from build123d import *

# Parameters (mm, degrees)
BOSS_EXTRUDE2_DEPTH     = 35
SKETCH2_R               = 11
CUT_EXTRUDE1_DEPTH      = 35
SKETCH3_R               = 1.4605
CUT_EXTRUDE2_DEPTH      = 4.064
CUT_EXTRUDE3_REACH      = 55.991
CUT_EXTRUDE3_END_RADIUS = 11
SKETCH4_R               = 1.4605
LPATTERN1_COUNT         = 7
LPATTERN1_PITCH         = 3.5


with BuildPart() as part:
    # Sketch1 → Boss-Extrude2 (new body)
    with BuildSketch(Plane.XY):
        with BuildLine():
            Line((-12.177746097, -15.45), (-5.620498199, 2.1))
            ThreePointArc((-5.620498199, 2.1), (0, 6), (5.620498199, 2.1))
            Line((5.620498199, 2.1), (12.177746097, -15.45))
            ThreePointArc((12.177746097, -15.45), (0, -33), (-12.177746097, -15.45))
        make_face()
    extrude(amount=-BOSS_EXTRUDE2_DEPTH)

    # Sketch2 → Cut-Extrude1 (cut)
    with BuildSketch(Plane.XY):
        with Locations((0, -20)):
            Circle(SKETCH2_R)
    extrude(amount=-CUT_EXTRUDE1_DEPTH, mode=Mode.SUBTRACT)

    # Sketch3 → Cut-Extrude2 (cut)
    with BuildSketch(Plane.XY):
        with Locations((0, -9)):
            Circle(SKETCH3_R)
    extrude(amount=-CUT_EXTRUDE2_DEPTH, mode=Mode.SUBTRACT)

    # Cut-Extrude3: up to this cylinder (the profile starts outside it)
    cut_extrude3_end = Plane(origin=(0, -20, -32.5), z_dir=(0, 0, 1)) * Cylinder(CUT_EXTRUDE3_END_RADIUS, 134.982, mode=Mode.PRIVATE)
    # Sketch4 → Cut-Extrude3 (cut, up to the surface)
    with BuildSketch(Plane(origin=(0, 6, 0), x_dir=(1, 0, 0), z_dir=(0, 1, 0)), mode=Mode.PRIVATE) as cut_extrude3_sk1:
        with Locations(Location((0, 32.5, 0), (0, 0, 270))):
            Circle(SKETCH4_R)
    cut_extrude3_tool1 = extrude(cut_extrude3_sk1.sketch, amount=-CUT_EXTRUDE3_REACH, mode=Mode.PRIVATE) - cut_extrude3_end
    cut_extrude3 = cut_extrude3_tool1.solids().sort_by_distance((0, 6, -32.5))[0]
    add(cut_extrude3, mode=Mode.SUBTRACT)

    # LPattern1: Cut-Extrude3 ×7
    with Locations(*[(0, 0, i * LPATTERN1_PITCH) for i in range(1, LPATTERN1_COUNT)]):
        add(cut_extrude3, mode=Mode.SUBTRACT)


solid = part.part
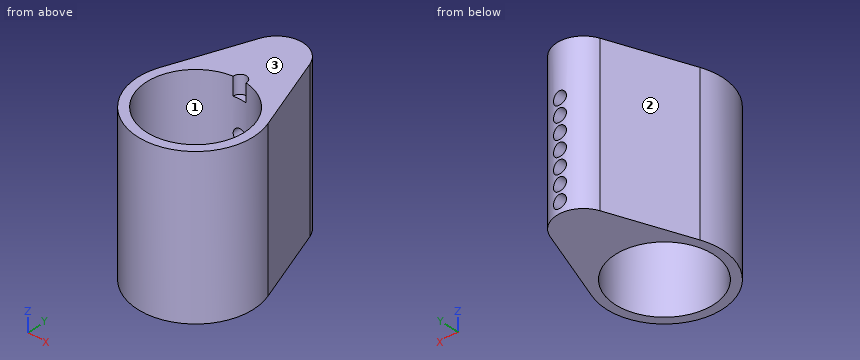
The listing builds one solid part. Answer for the finished solid, in the listing's coordinates (mm). Face numbers are marked on the shaded views. Coordinates: 2 decimals unless noted, no trailing zeros. Order: outer loops, then holes, each group sorted by start corner. A loop starts at its lowest first (then second) coordinate and runs counter-clockwise, first axis right, second up. Notation, with made-up numbers: M -15,-29.5 L 13,-29.5 A17 ccw 13,-5.5 Z; hole C 16.25,13.5 d4. An arc over 180 degrees is marked long. Use CSV: the item, a comma, the result in double quotes.
Q1. Given pin 1 Ø5 at (x, z) = (-3.5, -22.5) entering from +Y; pin 2 Ø2.5 at (x, z) = (0, -29) entering from +Y; pin 3 Ø1.8 at (x, z) = (0, -18.5) entering from +Y; pin 4 Ø3.5 at (x, z) = (0, -32.5) entering from +Y, each flat-ended and moving along its own axis, determine where each tip first touches the part or whether it passes through.
Here are the results:
pin 1,"y = 5.91"
pin 2,"y = -30.93"
pin 3,"y = -30.96"
pin 4,"y = 6"
Q2. Section B-B (x = -10) is taken. Determine the outline of the cut face in (y, z).
Here are the results:
outline,"M -28.31,-35 L -24.58,-35 L -24.58,0 L -28.31,0 Z; M -15.42,-35 L -9.62,-35 L -9.62,0 L -15.42,0 Z"
Q3. Section C-C (z = -8.5) is taken. Determine the outline of the cut face in (x, y).
Here are the results:
outline,"M -12.18,-15.45 A13 ccw long 12.18,-15.45 L 5.62,2.1 A6 ccw -5.62,2.1 Z; hole C 0,-20 d22"
Q4. Straight lines are drawn through the part: L1, parallel to X at y = -20.5, z = -6; L2, parallel to X at y = 0, z = -32; L3, parallel to Y at x = -3.75, z = -20.5. For each, find the intervals that lie inside material, in ascending order.
Here are the results:
L1,"-12.99 to -10.99, 10.99 to 12.99"
L2,"-6.41 to -1.37, 1.37 to 6.41"
L3,"-32.45 to -30.34, -9.66 to 4.68"
Q5. Section D-D (y = 0.5) is taken. Determine the outline of the cut face in (x, z).
Here are the results:
outline,"M -6.22,-35 L 6.22,-35 L 6.22,0 L -6.22,0 Z; hole C 0,-32.5 d2.92; hole C 0,-29 d2.92; hole C 0,-25.5 d2.92; hole C 0,-22 d2.92; hole C 0,-18.5 d2.92; hole C 0,-15 d2.92; hole C 0,-11.5 d2.92"
Q6. Section A-A (y = -20) is taken. Determine the outline of the cut face in (x, z), then the cut area to 3 significant figures.
Here are the results:
outline,"M -13,-35 L -11,-35 L -11,0 L -13,0 Z; M 11,-35 L 13,-35 L 13,0 L 11,0 Z"
area,"140 mm2"
Q7. Determine the mould class of the marked faces 1, 2 and 3 for opening direction X: pulls with the +X half, pulls with the -X half, needs draft (parallel to the pull), parting line crosses it, or undercut.
Here are the results:
face 1,"undercut"
face 2,"pulls with the -X half"
face 3,"needs draft"
